Work out the finished part from the listing and answer in its coordinate system (mm). A direction names the side the tool comes from. Give positions to 0.01 mm unless a question says otherwise; leave off trailing zeros. Write each loop counter-clockwise with the first axis right and the second up, starting at its lowest first coordinate (ties: lowest second). Pieces come first, ordered by that corner, then holes. Notation, with made-up numbers: (40, 87) -> (83, 87) arc R31 ccw to (83, 121) -> close; hole circle Ø10 at (15.25, 16.5). An arc over 180 degrees is marked (long way). Write item = value, one per line. Start each with the question number.
from build123d import *

# Parameters (mm, degrees)
SKETCH1_R           = 4
BOSS_EXTRUDE1_DEPTH = 4
SKETCH2_W           = 2
SKETCH2_H           = 10
BOSS_EXTRUDE2_DEPTH = 2
CHAMFER1_SIZE       = 1


with BuildPart() as part:
    # Sketch1 → Boss-Extrude1 (new body)
    with BuildSketch(Plane(origin=(0, 0, 0), x_dir=(1, 0, 0), z_dir=(0, 1, 0))):
        with Locations(Location((0, 0, 0), (0, 0, 270))):
            Circle(SKETCH1_R)
    extrude(amount=BOSS_EXTRUDE1_DEPTH)

    # Sketch2 → Boss-Extrude2 (add)
    with BuildSketch(Plane.XZ):
        Rectangle(SKETCH2_W, SKETCH2_H)
    extrude(amount=-BOSS_EXTRUDE2_DEPTH)

    # Chamfer1
    chamfer1_edges = [part.edges().sort_by_distance(p)[0] for p in [
        (0, 4, -4),
    ]]
    chamfer(chamfer1_edges, length=CHAMFER1_SIZE)


solid = part.part
(1) A cutting plane is placed at C-C, the plane y = 3.7. Write down the section's boundary in (x, z), then the cut area to 3 significant figures.
(2) A cutting plane is placed at B-B, the plane z = 0. Write down the section's boundary in (x, y), then the cut area to 3 significant figures.
(3) A cutting plane is placed at D-D, the plane z = 4.25. Write down the section's boundary in (x, y), then the cut area to 3 significant figures.
(4) For faces 4 (the flat face through (-1, 1, 4.4)), 5 (the flat face through (1, 1, 4.4)), 6 (the flat face through (1, 1, -4.4)), determine the directions among +Z, -Z, +X, -X, +Y, -Y from which every point of the face is accessible in a straight line to the end or side of a thin tool.
(5) Find the intervals of material crossed by line 1 along Y through (x, z) = (0.75, -4); line 2 along X through (y, z) = (0.95, 0.5); line 3 along X through (y, z) = (3.1, -1.75), in increasing order.
(6) Determine the mould class of faces 1 (the flat face through (0, 2, 4.4)), 2 (the flat face through (0, 0, 0)), 3 (the flat face through (-1, 1, -4.4)) for opening direction Y: pulls with the +Y half, pulls with the -Y half, needs draft (parallel to the pull), parting line crosses it, or undercut.
(7) A cutting plane is placed at A-A, the plane x = 0. Write down the section's boundary in (y, z).
(8) Each of these flat-tipped pins is pushed along its axis until it touches: pin 1 (1.5 mm diameter, centred on x = -1.5, z = 3.5, fed in from -Y); pin 2 (1.2 mm diameter, centred on y = 1, z = -4, fed in from +X); pin 3 (0.9 mm diameter, centred on x = 0, z = 4, fed in from +Y); pin 4 (0.6 mm diameter, centred on y = 1, z = 4.5, fed in from -X). Where does it stop, or does it pass through?
Results list:
q1.outline = circle Ø6.6 at (0, 0)
q1.area = 34.2 mm²
q2.outline = (-4, 0) -> (4, 0) -> (4, 3) -> (3, 4) -> (-3, 4) -> (-4, 3) -> close
q2.area = 31.0 mm²
q3.outline = (-1, 0) -> (1, 0) -> (1, 2) -> (-1, 2) -> close
q3.area = 4.00 mm²
q4.face_4 = +Z, -X, +Y, -Y
q4.face_5 = +Z, +X, +Y, -Y
q4.face_6 = -Z, +X, +Y, -Y
q5.line_1 = 0 to 2
q5.line_2 = -3.97 to 3.97
q5.line_3 = -3.49 to 3.49
q6.face_1 = pulls with the +Y half
q6.face_2 = pulls with the -Y half
q6.face_3 = needs draft
q7.outline = (0, -5) -> (2, -5) -> (2, -4) -> (3, -4) -> (4, -3) -> (4, 3) -> (3, 4) -> (2, 4) -> (2, 5) -> (0, 5) -> close
q8.pin_1 = 0
q8.pin_2 = 2.11
q8.pin_3 = 3.45
q8.pin_4 = -1
